Work out the finished part from the listing and answer in its coordinate system (mm). A direction names the side the tool comes from. Round coordinates to 2 decimals unless told otherwise and drop trailing zeros. Write each loop counter-clockwise with the first axis right and the second up, starting at its lowest first coordinate (ties: lowest second). Pieces come first, ordered by that corner, then holes.
from build123d import *

# Parameters (mm, degrees)
SKETCH1_R           = 3.5
BOSS_EXTRUDE1_DEPTH = 2.25
SKETCH2_R           = 5.5
BOSS_EXTRUDE2_DEPTH = 36.75
CUT_EXTRUDE1_START  = -33
SKETCH3_R           = 3.5
CUT_EXTRUDE1_DEPTH  = 33
CUT_EXTRUDE2_REACH  = 41.768
SKETCH4_R           = 2
CHAMFER1_SIZE2      = 1.5
CHAMFER1_SIZE       = 1
CUT_EXTRUDE3_DEPTH  = 40.76807765


with BuildPart() as part:
    # Sketch1 → Boss-Extrude1 (new body)
    with BuildSketch(Plane.XY):
        Circle(SKETCH1_R)
    extrude(amount=BOSS_EXTRUDE1_DEPTH)

    # Sketch2 → Boss-Extrude2 (add)
    with BuildSketch(Plane.XY.offset(2.25)):
        Circle(SKETCH2_R)
    extrude(amount=BOSS_EXTRUDE2_DEPTH)

    # Sketch3 → Cut-Extrude1 (cut)
    with BuildSketch(Plane.XY.offset(39).offset(CUT_EXTRUDE1_START)):
        Circle(SKETCH3_R)
    extrude(amount=CUT_EXTRUDE1_DEPTH, mode=Mode.SUBTRACT)

    # Sketch4 → Cut-Extrude2 (cut, up to next)
    with BuildSketch(Plane(origin=(0, 0, 0), x_dir=(-1, 0, 0), z_dir=(0, 0, -1)), mode=Mode.PRIVATE) as cut_extrude2_sk1:
        Circle(SKETCH4_R)
    cut_extrude2_tool1 = extrude(cut_extrude2_sk1.sketch, amount=-CUT_EXTRUDE2_REACH, mode=Mode.PRIVATE) & part.part
    add(cut_extrude2_tool1.solids().sort_by_distance((0, 0, 0))[0], mode=Mode.SUBTRACT)

    # Chamfer1
    chamfer1_edges = [part.edges().sort_by_distance(p)[0] for p in [
        (-3.5, 0, 6),
    ]]
    chamfer1_side = [part.faces().sort_by_distance(p)[0] for p in [
        (-3.5, 0, 6.02),
    ]]
    chamfer(chamfer1_edges, length=CHAMFER1_SIZE - 0.0001, length2=CHAMFER1_SIZE2 - 0.0001, reference=chamfer1_side[0])  # a hair under: the kernel refuses the full size

    # Sketch5 → Cut-Extrude3 (cut, through all)
    with BuildSketch(Plane(origin=(0, 0, 0), x_dir=(1, 0, 0), z_dir=(0, 1, 0))):
        with BuildLine():
            Line((-1.5, -11.5), (-1.5, -31.5))
            ThreePointArc((-1.5, -31.5), (0, -33), (1.5, -31.5))
            Line((1.5, -31.5), (1.5, -11.5))
            ThreePointArc((1.5, -11.5), (0, -10), (-1.5, -11.5))
        make_face()
    extrude(amount=CUT_EXTRUDE3_DEPTH, mode=Mode.SUBTRACT)


solid = part.part
Q1. A tool of negligible diameter and unlimited length cuts with its end or side. For faces 1 (the face through (3.233, -1.341, 1.109)), 2 (the face through (2, -2, 0)), 3 (the face through (0, 4, 10)), 4 (the face through (-0.759, -3.417, 22.776)), from which of +Z, -Z, +X, -X, +Y, -Y can it reach the whole face along a straight path? Write none if from no direction.
Q2. Given pin 1 (3 mm diameter, centred on x = -1, y = -0.5, fed in from +Z); pin 2 (5 mm diameter, centred on x = 0, y = 0, fed in from +Z); pin 3 (1.5 mm diameter, centred on y = -3, z = 13, fed in from +X); pin 4 (2 mm diameter, centred on x = 0, y = -0.5, fed in from -Z), each flat-ended and moving along its own axis, determine where each tip first touches the part or whether it passes through.
Q3. Find section D-D (y = -4). Determine the outline of the cut face in (x, z), plus the area to 3 significant figures.
Q4. Find section C-C (z = 19). Determine the outline of the cut face in (x, y), plus the area to 3 significant figures.
Q5. Find section A-A (x = 0). Count the separate pieces of the cut face and the enclosed holes in it, plus the area to 4 significant figures.
Q6. Find the intervals of material crossed by L1, parallel to Y at x = 0, z = 1.65; L2, parallel to Y at x = -0.25, z = 24; L3, parallel to Y at x = 3, z = 36.5, in increasing order.
Q7. The mould has two halves that part along Z. Classify faces 5 (the face through (-1.5, 4, 21)), 6 (the face through (4, 0, 39)), 7 (the face through (1.5, 4, 22)), 8 (the face through (4, 0, 2.25)): +Z half, -Z half, draft (parallel to the pull), parting line (faces both ways), or undercut.
Report:
1. face 1: -Z
1. face 2: -Z, +X, -X, +Y, -Y
1. face 3: +Y
1. face 4: +Z
2. pin 1: stops at z = 6.41
2. pin 2: stops at z = 6.33
2. pin 3: stops at x = 5.02
2. pin 4: passes through
3. outline: (-3.77, 2.25) - (3.77, 2.25) - (3.77, 39) - (-3.77, 39) - close
3. area: 277 mm2
4. outline: (-1.5, 3.16) - (-1.5, 5.29) arc R5.5 ccw (long way) to (1.5, 5.29) - (1.5, 3.16) arc R3.5 cw (long way) to start
4. area: 50.4 mm2
5. separate pieces: 3
5. enclosed holes: 0
5. area: 120.5 mm2
6. L1: y = -3.5 to -2, 2 to 3.5
6. L2: y = -5.49 to -3.49
6. L3: y = -4.61 to -1.8, 1.8 to 4.61
7. face 5: undercut
7. face 6: +Z half
7. face 7: undercut
7. face 8: -Z half
